Could you check a few things on this model? Use its own coordinates, in mm. Face numbers are marked on the shaded views. A direction names the side the tool comes from. Give positions to 0.01 mm unless a question says otherwise; leave off trailing zeros. Write each loop counter-clockwise with the first axis right and the second up, starting at its lowest first coordinate (ties: lowest second). Pieces come first, ordered by that corner, then holes. Notation, with made-up numbers: (-17.5, -39) - (-0.5, -39) arc R22 cw to (-0.5, -13) - close; hole circle Ø2 at (-14, 1.5). An arc over 180 degrees is marked (long way). Answer in a Markdown table with one row per item.
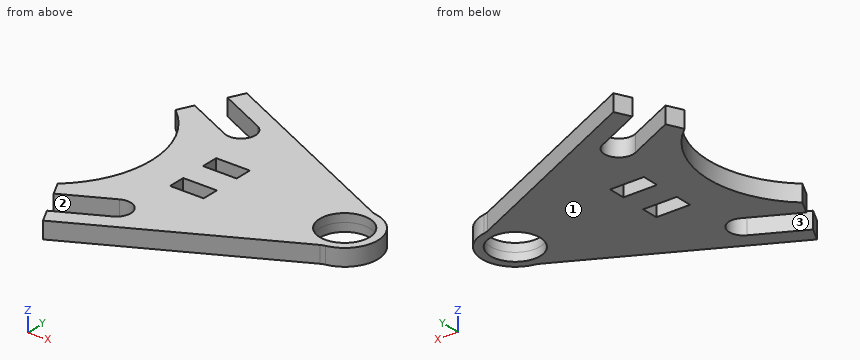
from build123d import *

# Parameters (mm, degrees)
SKETCH1_R           = 12.573
SKETCH1_R_2         = 9.398
BOSS_EXTRUDE1_DEPTH = 3.175
FILLET1_R           = 38.1
FILLET2_R           = 6.35
SKETCH2_W           = 12.7
SKETCH2_H           = 6.35
CUT_EXTRUDE1_DEPTH  = 3.175


with BuildPart() as part:
    # Sketch1 → Boss-Extrude1 (new, symmetric)
    # profile 1 of 4: a face of its own
    with BuildSketch(Plane.XY):
        with BuildLine():
            Line((503.446781124, -1524.922120572), (521.448925186, -1533.494549061))
            ThreePointArc((521.448925186, -1533.494549061), (524.031586139, -1540.772935173), (516.753200026, -1543.355596126))
            Line((516.753200026, -1543.355596126), (498.751055965, -1534.783167637))
            Line((498.751055965, -1534.783167637), (496.020983198, -1540.516334536))
            Line((496.020983198, -1540.516334536), (554.871597872, -1568.540367902))
            Line((554.871597872, -1568.540367902), (572.088750719, -1559.584617136))
            ThreePointArc((572.088750719, -1559.584617136), (576.84535815, -1556.340422204), (582.549387726, -1555.556737566))
            Line((582.549387726, -1555.556737566), (506.176853892, -1519.188953673))
            Line((506.176853892, -1519.188953673), (503.446781124, -1524.922120572))
        make_face()
    # profile 2 of 4: a face of its own
    with BuildSketch(Plane.XY):
        with BuildLine():
            ThreePointArc((572.393517032, -1576.884118428), (568.792205752, -1568.295127748), (572.088750719, -1559.584617136))
            Line((572.088750719, -1559.584617136), (554.871597872, -1568.540367902))
            Line((554.871597872, -1568.540367902), (572.393517032, -1576.884118428))
        make_face()
    # profile 3 of 4: a face of its own
    with BuildSketch(Plane.XY):
        with BuildLine():
            Line((572.393517032, -1576.884118428), (554.871597872, -1568.540367902))
            Line((554.871597872, -1568.540367902), (497.044597377, -1598.619917556))
            Line((497.044597377, -1598.619917556), (499.974916446, -1604.253365004))
            Line((499.974916446, -1604.253365004), (517.663941434, -1595.052163128))
            ThreePointArc((517.663941434, -1595.052163128), (525.028780639, -1597.376853534), (522.704090232, -1604.741692739))
            Line((522.704090232, -1604.741692739), (505.015065244, -1613.942894615))
            Line((505.015065244, -1613.942894615), (507.945384313, -1619.576342064))
            Line((507.945384313, -1619.576342064), (582.989537655, -1580.541041645))
            ThreePointArc((582.989537655, -1580.541041645), (577.261443726, -1579.958757387), (572.393517032, -1576.884118428))
        make_face()
    # profile 4 of 4: a face of its own
    with BuildSketch(Plane.XY):
        with Locations((581.363255123, -1568.073662845)):
            Circle(SKETCH1_R)
        with Locations((581.363255123, -1568.073662845)):
            Circle(SKETCH1_R_2, mode=Mode.SUBTRACT)
    extrude(amount=BOSS_EXTRUDE1_DEPTH, both=True)

    # Fillet1
    # the kernel refuses this fillet: 38.1 mm, written as the material it adds along each edge
    with BuildSketch(Plane(origin=(554.871597872, -1568.540367902, -3.175), x_dir=(-0.9028609288940066, 0.4299327192441295, 0), z_dir=(0, 0, 1))) as fillet1_piece_1:
        with BuildLine():
            CenterArc((74.290255, 36.995356759), FILLET1_R, 156.775740193, 99.393657747)
            Line((39.277556806, 52.01936971), (0, 0))
            Line((0, 0), (65.1823695, 0))
        make_face()
    extrude(amount=6.35)

    # Fillet2
    fillet2_edges = [part.edges().sort_by_distance(p)[0] for p in [
        (582.549387726, -1555.556737566, 0),
        (582.989537655, -1580.541041645, 0),
    ]]
    fillet(fillet2_edges, radius=FILLET2_R)

    # Sketch2 → Cut-Extrude1 (cut, symmetric)
    with BuildSketch(Plane.XY):
        with Locations((530.563255123, -1560.136162845)):
            Rectangle(SKETCH2_W, SKETCH2_H)
        with Locations((530.563255123, -1576.011162845)):
            Rectangle(SKETCH2_W, SKETCH2_H)
    extrude(amount=CUT_EXTRUDE1_DEPTH, both=True, mode=Mode.SUBTRACT)


solid = part.part
1) Imagine slicing it at D-D (y = -1538.5). List the corners of the cut face in (x, z) for me (3 decimals), then the cut area to 3 significant figures.
Check values:
| item | result |
|---|---|
| outline | (496.981, -3.175) - (506.556, -3.175) - (506.556, 3.175) - (496.981, 3.175) - close; (524.562, -3.175) - (546.73, -3.175) - (546.73, 3.175) - (524.562, 3.175) - close |
| area | 202 mm2 |
2) If I drill on line 1 (Y direction, x = 519, z = -3); line 2 (X direction, y = -1574.5, z = -3); line 3 (X direction, y = -1575.5, z = -1.5), over which ranges is the centre line in solid material (lowest first)?
Check values:
| item | result |
|---|---|
| line 1 | y = -1613.83 to -1606.67, -1594.57 to -1543.89, -1532.33 to -1525.3 |
| line 2 | x = 509.73 to 524.21, 536.91 to 574.51, 588.22 to 592.17 |
| line 3 | x = 509.59 to 524.21, 536.91 to 575.6, 587.12 to 591.51 |
3) Will these pins go through, and if not, where does the flat tip stop? P1, Ø1.9, axis at x = 531.5, z = 1.5, coming from the +Y side; P2, Ø5, axis at x = 576.5, y = -1571, coming from the -Z side; P3, Ø1.5, axis at x = 558.5, z = 0.5, coming from the +Y side; P4, Ø3, axis at x = 530.5, z = -1.5, coming from the -Y side.
Check values:
| item | result |
|---|---|
| P1 | stops at y = -1530.8 |
| P2 | passes through |
| P3 | stops at y = -1543.75 |
| P4 | stops at y = -1608.62 |
4) Imagine slicing it at B-B (y = -1574). List the corners of the cut face in (x, z) for me (3 decimals), then the cut area to 3 significant figures.
Check values:
| item | result |
|---|---|
| outline | (509.782, -3.175) - (524.213, -3.175) - (524.213, 3.175) - (509.782, 3.175) - close; (536.913, -3.175) - (574.069, -3.175) - (574.069, 3.175) - (536.913, 3.175) - close; (588.657, -3.175) - (592.452, -3.175) - (592.452, 3.175) - (588.657, 3.175) - close |
| area | 352 mm2 |
5) Imagine slicing it at C-C (x = 528). List the corners of the cut face in (y, z) for me (3 decimals).
Check values:
| item | result |
|---|---|
| outline | (-1609.145, -3.175) - (-1579.186, -3.175) - (-1579.186, 3.175) - (-1609.145, 3.175) - close; (-1572.836, -3.175) - (-1563.311, -3.175) - (-1563.311, 3.175) - (-1572.836, 3.175) - close; (-1556.961, -3.175) - (-1529.581, -3.175) - (-1529.581, 3.175) - (-1556.961, 3.175) - close |
6) On a 3-axis mill with a long thin cutter (end or side, diameter ignored), from which of +Z, -Z, +X, -X, +Y, -Y can I reach the whole of each face in a straight line? I mean the marked faces 1, 2 and 3. Say none if no direction works.
Check values:
| item | result |
|---|---|
| face 1 | -Z, +X, -X, +Y, -Y |
| face 2 | +Z, -Z |
| face 3 | +Z, -Z, -X |
7) Imagine slicing it at A-A (x = 577). List the corners of the cut face in (y, z) for me (3 decimals).
Check values:
| item | result |
|---|---|
| outline | (-1583.657, -3.175) - (-1576.397, -3.175) - (-1576.397, 3.175) - (-1583.657, 3.175) - close; (-1559.75, -3.175) - (-1552.914, -3.175) - (-1552.914, 3.175) - (-1559.75, 3.175) - close |
